from build123d import *

# Parameters (mm, degrees)
EXTRUDE_1_DEPTH     = 60
FILLET_1_R          = 5
SKETCH_3_R          = 2.5
CUT_EXTRUDE_2_DEPTH = 77.472217177
CUT_EXTRUDE_4_DEPTH = 6
SKETCH_6_W          = 18
SKETCH_6_H          = 20
CUT_EXTRUDE_5_DEPTH = 5.9
SKETCH_7_R          = 2.5
EXTRUDE_2_DEPTH     = 5
CUT_EXTRUDE_START   = -8
CUT_EXTRUDE_6_DEPTH = 8
EXTRUDE_3_DEPTH     = 5
EXTRUDE_4_DEPTH     = 5
EXTRUDE_5_DEPTH     = 45
CUT_EXTRUDE_7_DEPTH = 15


with BuildPart() as part:
    # Sketch 1 → Extrude 1 (new body)
    with BuildSketch(Plane.XY):
        Polygon((0, 9), (0, -11), (42, -11), (42, 11), (40.535898385, 9), (40, 11), (38.535898385, 9), (38, 11), (36.535898385, 9), (36, 11), (34.535898385, 9), (34, 11), (32.535898385, 9), (32, 11), (30.535898385, 9), (30, 11), (28.535898385, 9), (28, 11), (26.535898385, 9), (26, 11), (24.535898385, 9), (24, 11), (22.535898385, 9), (22, 11), (20.535898385, 9), (20, 11), (18.535898385, 9), (18, 11), (16.535898385, 9), (16, 11), (14.535898385, 9), (14, 11), (12.535898385, 9), (12, 11), (10.535898385, 9), (10, 11), (8.51763809, 9.068148347), (8, 11), (6, 9), align=None)
    extrude(amount=EXTRUDE_1_DEPTH)

    # Fillet 1
    fillet_1_edges = [part.edges().sort_by_distance(p)[0] for p in [
        (42, 0, 0),
        (42, 0, 60),
    ]]
    fillet(fillet_1_edges, radius=FILLET_1_R)

    # Sketch 3 → Cut-Extrude 2 (cut, through all)
    with BuildSketch(Plane.XZ.offset(11)):
        with Locations(Location((30, 8, 0), (0, 0, 270))):
            Circle(SKETCH_3_R)
        with BuildLine():
            ThreePointArc((14.7, 52), (13.967766953, 53.767766953), (12.2, 54.5))
            Line((12.2, 54.5), (12.2, 49.5))
            ThreePointArc((12.2, 49.5), (13.967766953, 50.232233047), (14.7, 52))
        make_face()
        with BuildLine():
            Line((12.2, 49.5), (12.2, 54.5))
            ThreePointArc((12.2, 54.5), (9.7, 52), (12.2, 49.5))
        make_face()
        with BuildLine():
            ThreePointArc((14.7, 8), (13.967766953, 9.767766953), (12.2, 10.5))
            Line((12.2, 10.5), (12.2, 5.5))
            ThreePointArc((12.2, 5.5), (13.967766953, 6.232233047), (14.7, 8))
        make_face()
        with BuildLine():
            Line((12.2, 5.5), (12.2, 10.5))
            ThreePointArc((12.2, 10.5), (9.7, 8), (12.2, 5.5))
        make_face()
        with Locations(Location((30, 52, 0), (0, 0, 270))):
            Circle(SKETCH_3_R)
    extrude(amount=-CUT_EXTRUDE_2_DEPTH, mode=Mode.SUBTRACT)

    # Sketch 5 → Cut-Extrude 4 (cut)
    with BuildSketch(Plane.ZY):
        with BuildLine():
            Line((27.05, 9), (32.95, 9))
            ThreePointArc((32.95, 9), (30, 6.05), (27.05, 9))
        make_face()
    extrude(amount=-CUT_EXTRUDE_4_DEPTH, mode=Mode.SUBTRACT)

    # Sketch 6 → Cut-Extrude 5 (cut)
    with BuildSketch(Plane.ZY):
        with Locations((30, -1)):
            Rectangle(SKETCH_6_W, SKETCH_6_H)
    extrude(amount=-CUT_EXTRUDE_5_DEPTH, mode=Mode.SUBTRACT)

    # Sketch 8 → Cut-Extrude 6 (cut)
    with BuildSketch(Plane.XZ.offset(11).offset(CUT_EXTRUDE_START)):
        with BuildLine():
            Line((6, 60), (6, 0))
            Line((6, 0), (37, 0))
            ThreePointArc((37, 0), (40.535533906, 1.464466094), (42, 5))
            Line((42, 5), (42, 55))
            ThreePointArc((42, 55), (40.535533906, 58.535533906), (37, 60))
            Line((37, 60), (6, 60))
        make_face()
    extrude(amount=CUT_EXTRUDE_6_DEPTH, mode=Mode.SUBTRACT)



with BuildPart() as body_2:
    # Sketch 7 → Extrude 2 (new body)
    # profile 1 of 3: a face of its own
    with BuildSketch(Plane.XZ.offset(11)):
        Polygon((0, 39), (0, 60), (-19, 60), (-19, 0), (0, 0), (0, 21), (5.9, 21), (5.9, 30), (5.9, 39), align=None)
        with Locations((-7, 14)):
            Circle(SKETCH_7_R, mode=Mode.SUBTRACT)
        with Locations((-7, 46)):
            Circle(SKETCH_7_R, mode=Mode.SUBTRACT)
    # profile 2 of 3: a face of its own
    with BuildSketch(Plane.XZ.offset(11)):
        Polygon((6, 30), (6, 60), (0, 60), (0, 39), (5.9, 39), (5.9, 30), align=None)
    # profile 3 of 3: a face of its own
    with BuildSketch(Plane.XZ.offset(11)):
        Polygon((6, 0), (6, 30), (5.9, 30), (5.9, 21), (0, 21), (0, 0), align=None)
    extrude(amount=EXTRUDE_2_DEPTH)


with BuildPart() as part_1:
    add(part.part)

    add(body_2.part)  # Extrude 3 merges body 2
    # Sketch 9 → Extrude 3 (add)
    with BuildSketch(Plane.XY.offset(60)):
        Polygon((0, 9), (-19, -11), (0, -11), align=None)
    extrude(amount=-EXTRUDE_3_DEPTH)

    # Sketch 10 → Extrude 4 (add)
    with BuildSketch(Plane(origin=(0, 0, 0), x_dir=(-1, 0, 0), z_dir=(0, 0, -1))):
        Polygon((0, 9), (0, -11), (19, -11), align=None)
    extrude(amount=-EXTRUDE_4_DEPTH)

    # Sketch 11 → Extrude 5 (add)
    with BuildSketch(Plane.XY.offset(60)):
        Polygon((6, -3), (6, -16), (37, -3), align=None)
    extrude(amount=-EXTRUDE_5_DEPTH)

    # Sketch 12 → Cut-Extrude 7 (cut)
    with BuildSketch(Plane.XY.offset(60)):
        Polygon((37, -3), (6, -3), (6, -16), align=None)
    extrude(amount=-CUT_EXTRUDE_7_DEPTH, mode=Mode.SUBTRACT)


solid = part_1.part
Here's how the part is built. I have some questions about the finished solid (model axes, mm). A direction names the side the tool comes from. Coordinates: 2 decimals unless noted, no trailing zeros. Order: outer loops, then holes, each group sorted by start corner. A loop starts at its lowest first (then second) coordinate and runs counter-clockwise, first axis right, second up. Notation, with made-up numbers: (84.25, 62.25) - (138.25, 62.25) arc R26 cw to (138.25, 81.25) - close; hole circle Ø3 at (51.5, -1.5). An arc over 180 degrees is marked (long way). Use CSV: the item, a comma, the result in double quotes. Start each with the question number.
1. Suppose I cut it at B-B on y = -0.75. List the corners of the cut face in (x, z) for me, then the cut area to 3 significant figures.
2. Suppose I cut it at C-C on y = -7.5. List the corners of the cut face in (x, z) for me (3 decimals).
3. Please list where these lines run through material, in increasing order: line 1 (X direction, y = 4.5, z = 52); line 2 (Z direction, x = -7, y = -12.65); line 3 (Z direction, x = 5.5, y = 8). Write a range as from..to.
4. Suppose I cut it at D-D on y = 3.5. List the corners of the cut face in (x, z) for me (3 decimals).
5. I'm going to push flat-ended pins straight in: pin 1 (6.5 mm diameter, centred on x = 3, z = 42, fed in from +Y); pin 2 (8 mm diameter, centred on y = -1, z = 46, fed in from -X); pin 3 (3 mm diameter, centred on y = 5.5, z = 27, fed in from -X). Where does each tip first touch, or does it pass through?
6. If we mould it in two halves opening along X, with no side actions, what happens to faces 1 (the face through (6, 8, 30)), 2 (the face through (12.27, 9.99, 2.72)), 3 (the face through (40, -3, 30))? For each: +X half, -X half, draft (parallel to the pull), parting line (faces both ways), or undercut.
7. For faces 4 (the face through (-5.85, -13.46, 11.78)), 5 (the face through (5.9, -1, 30)), which set-ups out of +Z, -Z, +X, -X, +Y, -Y let a thin tool reach every point of the face, with its end or its side?
8. Suppose I cut it at A-A on x = -7. List the corners of the cut face in (y, z) for me, then the cut area to 3 significant figures.
Output:
1,outline,"(-9.26, 0) - (37, 0) arc R5 ccw to (42, 5) - (42, 55) arc R5 ccw to (37, 60) - (-9.26, 60) - (-9.26, 55) - (0, 55) - (0, 39) - (5.9, 39) - (5.9, 21) - (0, 21) - (0, 5) - (-9.26, 5) - close; hole circle Ø5 at (12.2, 8); hole circle Ø5 at (12.2, 52); hole circle Ø5 at (30, 8); hole circle Ø5 at (30, 52)"
1,area,"2,420 mm2"
2,outline,"(-15.675, 0) - (6, 0) - (6, 15) - (26.269, 15) - (26.269, 45) - (6, 45) - (6, 60) - (-15.675, 60) - (-15.675, 55) - (0, 55) - (0, 39) - (5.9, 39) - (5.9, 21) - (0, 21) - (0, 5) - (-15.675, 5) - close"
3,line 1,"x = 0..9.7, 14.7..27.5, 32.5..42"
3,line 2,"z = 0..11.5, 16.5..43.5, 48.5..60"
3,line 3,"z = 0..21, 39..60"
4,outline,"(-5.225, 0) - (37, 0) arc R5 ccw to (42, 5) - (42, 55) arc R5 ccw to (37, 60) - (-5.225, 60) - (-5.225, 55) - (0, 55) - (0, 39) - (5.9, 39) - (5.9, 21) - (0, 21) - (0, 5) - (-5.225, 5) - close; hole circle Ø5 at (12.2, 8); hole circle Ø5 at (12.2, 52); hole circle Ø5 at (30, 8); hole circle Ø5 at (30, 52)"
5,pin 1,"stops at y = 9.25"
5,pin 2,"stops at x = 0"
5,pin 3,"stops at x = 5.9"
6,face 1,"-X half"
6,face 2,"undercut"
6,face 3,"draft"
7,face 4,"+Y, -Y"
7,face 5,"-X, +Y"
8,outline,"(-16, 0) - (1.63, 0) - (1.63, 5) - (-11, 5) - (-11, 11.5) - (-16, 11.5) - close; (-16, 16.5) - (-11, 16.5) - (-11, 43.5) - (-16, 43.5) - close; (-16, 48.5) - (-11, 48.5) - (-11, 55) - (1.63, 55) - (1.63, 60) - (-16, 60) - close"
8,area,"376 mm2"
